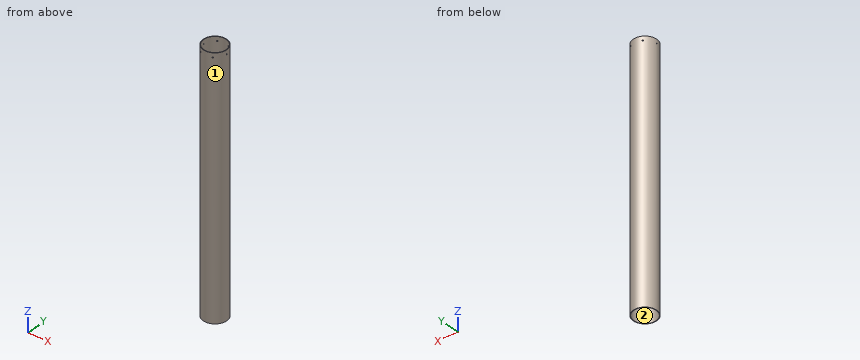
```python
from build123d import *

# Parameters (mm, degrees)
SKETCH3_R           = 42
SKETCH3_R_2         = 40
BOSS_EXTRUDE1_DEPTH = 910
CUT_EXTRUDE1_START  = -2.050031
SKETCH4_R           = 2
CUT_EXTRUDE1_DEPTH  = 2.050031
CIRPATTERN1_COUNT   = 6


with BuildPart() as part:
    # Sketch3 → Boss-Extrude1 (new body)
    with BuildSketch(Plane.XY.offset(455)):
        Circle(SKETCH3_R)
        Circle(SKETCH3_R_2, mode=Mode.SUBTRACT)
    extrude(amount=-BOSS_EXTRUDE1_DEPTH)

    # Sketch4 → Cut-Extrude1 (cut)
    with BuildSketch(Plane(origin=(42, 0, 0), x_dir=(0, 0, -1), z_dir=(1, 0, 0)).offset(CUT_EXTRUDE1_START)):
        with Locations((-440, 0)):
            Circle(SKETCH4_R)
    cut_extrude1 = extrude(amount=CUT_EXTRUDE1_DEPTH, mode=Mode.SUBTRACT)

    # CirPattern1: Cut-Extrude1 ×6 about axis
    cirpattern1_axis = Axis((0, 0, 455), (0, 0, 1))
    for i in range(1, CIRPATTERN1_COUNT):
        add(cut_extrude1.rotate(cirpattern1_axis, i * 360 / CIRPATTERN1_COUNT), mode=Mode.SUBTRACT)


solid = part.part
```
Check sheet for the modelled part. Datum: model origin and axes. Units: mm. Face numbers are marked on the shaded views. Coordinates: 2 decimals unless noted, no trailing zeros. Loops run counter-clockwise (first coordinate to the right, second up) from the corner with the lowest first, then second, coordinate; pieces in that order, holes last.
1) Gauge pin test, flat ends, axial feed: pin 1 (4 mm diameter, centred on y = -31.5, z = -160, fed in from +X); pin 2 (4 mm diameter, centred on x = 17, z = -115.5, fed in from -Y); pin 3 (1 mm diameter, centred on x = -21, z = -69, fed in from +Y). Record the tip position at first contact, or that the pin passes through.
2) Sectioned sample at B-B (y = -21). Record the boundary of the cut face in (x, z).
3) Release check for a two-part mould opening along Y. For the marked faces 1 and 2 record: released by +Y, released by -Y, zero draft, split by the parting line, or undercut.
4) Material ranges on probe 1 along Z at (x, y) = (40.75, 0); probe 2 along X at (y, z) = (2.5, 96); probe 3 along X at (y, z) = (-26.5, 266.5), recorded low to high.
5) Sectioned sample at A-A (x = 0). Record the boundary of the cut face in (y, z), and give its area (3 significant figures).
6) Sectioned sample at C-C (z = -376.5). Record the boundary of the cut face in (x, y).
Check sheet entries:
1. pin 1: stops at x = 29.9
1. pin 2: stops at y = -39.23
1. pin 3: stops at y = 36.66
2. outline: (-36.37, -455) - (-34.04, -455) - (-34.04, 455) - (-36.37, 455) - close; (34.04, -455) - (36.37, -455) - (36.37, 455) - (34.04, 455) - close
3. face 1: split by the parting line
3. face 2: undercut
4. probe 1: z = -455 to 438, 442 to 455
4. probe 2: x = -41.93 to -39.92, 39.92 to 41.93
4. probe 3: x = -32.58 to -29.96, 29.96 to 32.58
5. outline: (-42, -455) - (-40, -455) - (-40, 455) - (-42, 455) - close; (40, -455) - (42, -455) - (42, 455) - (40, 455) - close
5. area: 3,640 mm2
6. outline: circle Ø84 at (0, 0); hole circle Ø80 at (0, 0)
